Geometry: see drawing. Coordinates: mm, zero at the bounding-box minimum. Round coordinates to 2 decimals unless told otherwise and drop trailing zeros. Loops run counter-clockwise (first coordinate to the right, second up) from the corner with the lowest first, then second, coordinate; pieces in that order, holes last. Notation, with made-up numbers: (3.25, 26) - (14.25, 26) arc R12 cw to (14.25, 40) - close; hole circle Ø5 at (-11, -25.5). An arc over 180 degrees is marked (long way). Return JSON: item names as keys, results as strings. Group by question number.
1. Draft query along Y for the marked faces 1, 2 and 3. Return one class per face: +Y half, -Y half, draft (parallel to the pull), parting line (faces both ways), or undercut.
2. Section C-C on z = 5.45. Return loops of the section in (x, y).
3. Section B-B on y = 6.3. Return loops of the section in (x, z).
4. Section A-A on x = 24. Return loops of the section in (y, z), and give its area (3 significant figures).
5. Material intervals for probe 1 along Y at (x, z) = (6, 4.4); probe 2 along X at (y, z) = (45.5, 0.4); probe 3 along Y at (x, z) = (25.75, 4.85), sorted ascending.
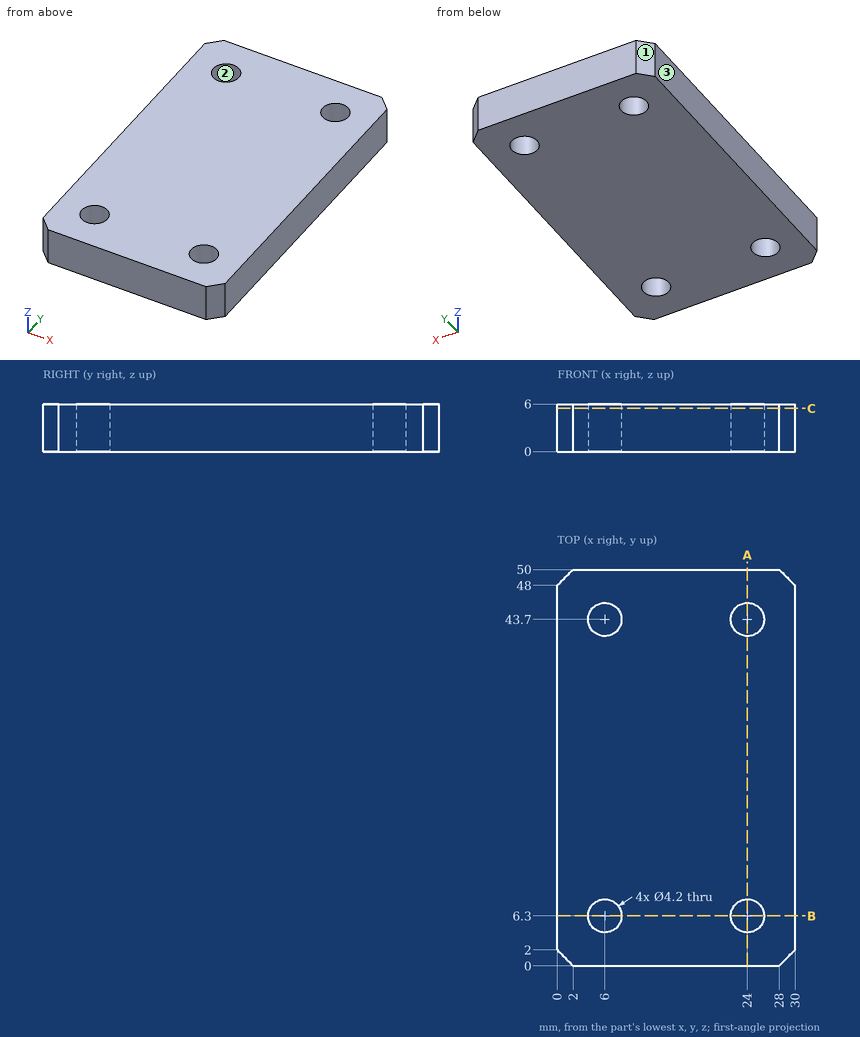
Taken from the geometry:
{
 "1": {"face 1": "+Y half", "face 2": "undercut", "face 3": "draft"},
 "2": {"outline": "(0, 2) - (2, 0) - (28, 0) - (30, 2) - (30, 48) - (28, 50) - (2, 50) - (0, 48) - close; hole circle Ø4.2 at (6, 6.3); hole circle Ø4.2 at (6, 43.7); hole circle Ø4.2 at (24, 6.3); hole circle Ø4.2 at (24, 43.7)"},
 "3": {"outline": "(0, 0) - (3.9, 0) - (3.9, 6) - (0, 6) - close; (8.1, 0) - (21.9, 0) - (21.9, 6) - (8.1, 6) - close; (26.1, 0) - (30, 0) - (30, 6) - (26.1, 6) - close"},
 "4": {"outline": "(0, 0) - (4.2, 0) - (4.2, 6) - (0, 6) - close; (8.4, 0) - (41.6, 0) - (41.6, 6) - (8.4, 6) - close; (45.8, 0) - (50, 0) - (50, 6) - (45.8, 6) - close", "area": "250 mm2"},
 "5": {"probe 1": "0 to 4.2, 8.4 to 41.6, 45.8 to 50", "probe 2": "0 to 4.92, 7.08 to 22.92, 25.08 to 30", "probe 3": "0 to 5.14, 7.46 to 42.54, 44.86 to 50"}
}
